```python
from build123d import *

# Parameters (mm, degrees)
BOSS_EXTRUDE1_DEPTH      = 3
BOSS_EXTRUDE1_DEPTH_BACK = 3
CUT_EXTRUDE1_DEPTH       = 77.793105304
CUT_EXTRUDE1_DEPTH_BACK  = 77.793105304
SKETCH2_R                = 1.375
FILLET2_R                = 3


with BuildPart() as part:
    # Sketch1 → Boss-Extrude1 (new, two sides: drawn at the far end of the back side and taken through both)
    with BuildSketch(Plane(origin=(0, 0, 0), x_dir=(1, 0, 0), z_dir=(0, 1, 0)).offset(-BOSS_EXTRUDE1_DEPTH_BACK)):
        Polygon((0, 41.898993428), (-49.75, -2.75), (-56.75, -2.75), (-56.75, -9.75), (-49.75, -9.75), (0, -29.761006572), (6.321904272, -29.761006572), (6.321904272, -20.181495095), (0, -20.181495095), (-8.267104031, -16.856207194), (-8.267104031, 24.303580089), (0, 31.723034833), (6.321904272, 31.723034833), (6.321904272, 41.898993428), align=None)
        with BuildLine():
            Line((-38.84115752, -6.072372844), (-38.84115752, -0.855123784))
            ThreePointArc((-38.84115752, -0.855123784), (-34.127327229, 0.958977223), (-29.413496938, -0.855123784))
            Line((-29.413496938, -0.855123784), (-29.413496938, -6.072372844))
            ThreePointArc((-29.413496938, -6.072372844), (-34.127327229, -7.886473851), (-38.84115752, -6.072372844))
        make_face(mode=Mode.SUBTRACT)
    extrude(amount=BOSS_EXTRUDE1_DEPTH + BOSS_EXTRUDE1_DEPTH_BACK)

    # Sketch2 → Cut-Extrude1 (cut, two sides: drawn at the far end of the back side and taken through both)
    with BuildSketch(Plane.XY.offset(9.75).offset(-CUT_EXTRUDE1_DEPTH_BACK)):
        with Locations((-53.75, 0)):
            Circle(SKETCH2_R)
        with Locations((3.321904272, 0)):
            Circle(SKETCH2_R)
        with BuildLine():
            Line((-53.75, -3), (-53.75, -4.40506942))
            Line((-53.75, -4.40506942), (3.321904272, -4.40506942))
            Line((3.321904272, -4.40506942), (3.321904272, -3))
            ThreePointArc((3.321904272, -3), (2.013077646, -2.699439361), (0.966505531, -1.857981908))
            ThreePointArc((0.966505531, -1.857981908), (0.3635922, -1.473684928), (-0.338629648, -1.339248585))
            Line((-0.338629648, -1.339248585), (-50.08946608, -1.339248585))
            ThreePointArc((-50.08946608, -1.339248585), (-50.791687928, -1.473684928), (-51.394601259, -1.857981908))
            ThreePointArc((-51.394601259, -1.857981908), (-52.441173374, -2.699439361), (-53.75, -3))
        make_face()
        with BuildLine():
            Line((3.321904272, 3), (3.321904272, 4.40506942))
            Line((3.321904272, 4.40506942), (-53.75, 4.40506942))
            Line((-53.75, 4.40506942), (-53.75, 3))
            ThreePointArc((-53.75, 3), (-52.441173374, 2.699439361), (-51.394601259, 1.857981908))
            ThreePointArc((-51.394601259, 1.857981908), (-50.791687928, 1.473684928), (-50.08946608, 1.339248585))
            Line((-50.08946608, 1.339248585), (-0.338629648, 1.339248585))
            ThreePointArc((-0.338629648, 1.339248585), (0.3635922, 1.473684928), (0.966505531, 1.857981908))
            ThreePointArc((0.966505531, 1.857981908), (2.013077646, 2.699439361), (3.321904272, 3))
        make_face()
    extrude(amount=CUT_EXTRUDE1_DEPTH + CUT_EXTRUDE1_DEPTH_BACK, mode=Mode.SUBTRACT)

    # Fillet2
    fillet2_edges = [part.edges().sort_by_distance(p)[0] for p in [
        (6.321904272, 3, -36.811014131),
        (6.321904272, -3, -36.811014131),
        (6.321904272, -3, 24.971250833),
        (6.321904272, 3, 24.971250833),
        (-56.75, -3, 6.25),
        (-56.75, 3, 6.25),
    ]]
    fillet(fillet2_edges, radius=FILLET2_R - 0.0001)  # a hair under: the kernel refuses the full size

    # Sketch3 → Revolve1 (revolve)
    with BuildSketch(Plane(origin=(0, 0, 0), x_dir=(1, 0, 0), z_dir=(0, 1, 0)), mode=Mode.PRIVATE) as revolve1_sk:
        with BuildLine():
            Line((-34.127327229, 0.958977223), (-33.377327229, 0.958977223))
            Line((-33.377327229, 0.958977223), (-33.377327229, -1.609698692))
            ThreePointArc((-33.377327229, -1.609698692), (-32.127327229, -3.463748314), (-33.377327229, -5.317797935))
            Line((-33.377327229, -5.317797935), (-33.377327229, -7.886473851))
            Line((-33.377327229, -7.886473851), (-34.127327229, -7.886473851))
            Line((-34.127327229, -7.886473851), (-34.127327229, 0.958977223))
        make_face()
    revolve(revolve1_sk.sketch.rotate(Axis((-34.127327229, 0, -0.958977223), (0, 0, 1)), 270), axis=Axis((-34.127327229, 0, -0.958977223), (0, 0, 1)))


solid = part.part
```
Read the model definition and answer for the solid it produces. Units are mm, in the model's axes. A direction names the side the tool comes from. Coordinates: 2 decimals unless noted, no trailing zeros. Order: outer loops, then holes, each group sorted by start corner. A loop starts at its lowest first (then second) coordinate and runs counter-clockwise, first axis right, second up. Notation, with made-up numbers: (76, -16.5) - (105, -16.5) arc R19 ccw to (105, 4.5) - close; hole circle Ø1 at (80, -2). An arc over 180 degrees is marked (long way). Answer as a JSON object with one key per item and string values. Group by question number.
Item 1: Flat-ended cylindrical pins translate along their axes: P1, Ø2, axis at x = 3.32, y = 0, coming from the -Z side; P2, Ø0.8, axis at y = -0.5, z = 6, coming from the +X side; P3, Ø3, axis at x = -9, z = 22.5, coming from the -Y side; P4, Ø1.8, axis at x = -52, y = 0, coming from the +Z side. Find the tip coordinate at first contact, or state that the pin passes through.
Item 2: Section A-A (x = -4) is taken. Give the vertices of the cut face in (y, z).
Item 3: A tool of negligible diameter and unlimited length cuts with its end or side. For faces 5 (the face through (-33.495, -0.403, 6.62)), 6 (the face through (-29.413, 0, 3)), 7 (the face through (-4.19, -0.02, -27.96)), from which of +Z, -Z, +X, -X, +Y, -Y can it reach the whole face along a straight path? Write none if from no direction.
Item 4: Consider probe 1 along Z at (x, y) = (-54, -2); probe 2 along Y at (x, z) = (-11, -22); probe 3 along Z at (x, y) = (-6, -0.5). Determine where each line is inside the solid, lowest interval first. Write a range as from..to.
Item 5: Section C-C (x = -47) is taken. Give the vertices of the cut face in (y, z), plus the area to 3 significant figures.
Item 6: The mould has two halves that part along X. Classify faces 1 (the face through (1.996, 2.691, -36.882)), 2 (the face through (-34.055, -0.912, 7.886)), 3 (the face through (-33.495, -0.403, 0.343)), 4 (the face through (-4.08, -0.02, 18.54)): +X half, -X half, draft (parallel to the pull), parting line (faces both ways), or undercut.
Results are:
{
 "1": {"P1": "passes through", "P2": "stops at x = -8.27", "P3": "stops at y = -1.34", "P4": "stops at z = 9.75"},
 "2": {"outline": "(-1.34, -38.31) - (1.34, -38.31) - (1.34, -28.13) - (-1.34, -28.13) - close; (-1.34, 18.57) - (1.34, 18.57) - (1.34, 28.15) - (-1.34, 28.15) - close"},
 "3": {"face 5": "none", "face 6": "+Y, -Y", "face 7": "+X, +Y, -Y"},
 "4": {"probe 1": "z = 2.75..9.75", "probe 2": "y = -1.34..1.34", "probe 3": "z = -36.51..-26.34, 17.77..27.35"},
 "5": {"outline": "(-1.34, 0.28) - (1.34, 0.28) - (1.34, 10.86) - (-1.34, 10.86) - close", "area": "28.3 mm^2"},
 "6": {"face 1": "-X half", "face 2": "undercut", "face 3": "undercut", "face 4": "+X half"}
}
